```python
from build123d import *

# Parameters (mm, degrees)
ESQUISSE1_W             = 180
ESQUISSE1_H             = 70
BOSS_EXTRU_1_DEPTH      = 5
ESQUISSE3_W             = 5
ESQUISSE3_H             = 10
ESQUISSE3_W_2           = 20
ESQUISSE3_H_2           = 5
ENL_V_MAT_EXTRU_2_DEPTH = 5
ESQUISSE4_W             = 2
ESQUISSE4_H             = 30
ENL_V_MAT_EXTRU_3_DEPTH = 5


with BuildPart() as part:
    # Esquisse1 → Boss.-Extru.1 (new body)
    with BuildSketch(Plane(origin=(0, 0, 0), x_dir=(0, 0, -1), z_dir=(1, 0, 0))):
        Rectangle(ESQUISSE1_W, ESQUISSE1_H)
    extrude(amount=BOSS_EXTRU_1_DEPTH)

    # Esquisse3 → Enlèv. mat.-Extru.2 (cut)
    with BuildSketch(Plane(origin=(5, 0, 0), x_dir=(0, 0, -1), z_dir=(1, 0, 0))):
        with Locations((-87.5, 30)):
            Rectangle(ESQUISSE3_W, ESQUISSE3_H)
        with Locations((-87.5, 5)):
            Rectangle(ESQUISSE3_W, ESQUISSE3_H)
        with Locations((87.5, 30)):
            Rectangle(ESQUISSE3_W, ESQUISSE3_H)
        with Locations((87.5, 5)):
            Rectangle(ESQUISSE3_W, ESQUISSE3_H)
        with Locations((-40, 32.5)):
            Rectangle(ESQUISSE3_W_2, ESQUISSE3_H_2)
        with Locations((40, 32.5)):
            Rectangle(ESQUISSE3_W_2, ESQUISSE3_H_2)
        with Locations((0, 32.5)):
            Rectangle(ESQUISSE3_W_2, ESQUISSE3_H_2)
        with Locations((-40, -32.5)):
            Rectangle(ESQUISSE3_W_2, ESQUISSE3_H_2)
        with Locations((0, -32.5)):
            Rectangle(ESQUISSE3_W_2, ESQUISSE3_H_2)
        with Locations((40, -32.5)):
            Rectangle(ESQUISSE3_W_2, ESQUISSE3_H_2)
    extrude(amount=-ENL_V_MAT_EXTRU_2_DEPTH, mode=Mode.SUBTRACT)

    # Esquisse4 → Enlèv. mat.-Extru.3 (cut)
    with BuildSketch(Plane(origin=(5, 0, 0), x_dir=(0, 0, -1), z_dir=(1, 0, 0))):
        with Locations((32, 5)):
            Rectangle(ESQUISSE4_W, ESQUISSE4_H)
        with Locations((39, 5)):
            Rectangle(ESQUISSE4_W, ESQUISSE4_H)
        with Locations((25, 5)):
            Rectangle(ESQUISSE4_W, ESQUISSE4_H)
        with Locations((18, 5)):
            Rectangle(ESQUISSE4_W, ESQUISSE4_H)
        with Locations((11, 5)):
            Rectangle(ESQUISSE4_W, ESQUISSE4_H)
        with Locations((4, 5)):
            Rectangle(ESQUISSE4_W, ESQUISSE4_H)
        with Locations((-3, 5)):
            Rectangle(ESQUISSE4_W, ESQUISSE4_H)
        with Locations((-10, 5)):
            Rectangle(ESQUISSE4_W, ESQUISSE4_H)
        with Locations((-17, 5)):
            Rectangle(ESQUISSE4_W, ESQUISSE4_H)
        with Locations((-24, 5)):
            Rectangle(ESQUISSE4_W, ESQUISSE4_H)
    extrude(amount=-ENL_V_MAT_EXTRU_3_DEPTH, mode=Mode.SUBTRACT)


solid = part.part
```
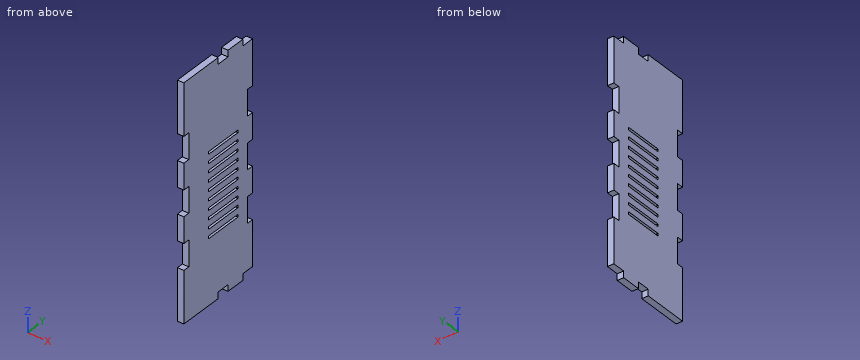
Geometry check sheet. Reference: the model listing, model coordinates, mm. Give positions to 0.01 mm unless a question says otherwise; leave off trailing zeros. Write each loop counter-clockwise with the first axis right and the second up, starting at its lowest first coordinate (ties: lowest second). Pieces come first, ordered by that corner, then holes. Notation, with made-up numbers: (-22.75, -21) -> (34.25, -21) arc R30 cw to (34.25, 3) -> close; hole circle Ø11 at (48.25, -1.75). An arc over 180 degrees is marked (long way). One line per question, with ' | ' between items.
Item 1: Depth check by flat-ended pin: pin 1 (2 mm diameter, centred on x = 2.5, z = -32, fed in from +Y); pin 2 (1.6 mm diameter, centred on x = 3.5, z = -4.5, fed in from -Y); pin 3 (2.5 mm diameter, centred on x = 3.5, y = 5.5, fed in from -Z). Enter the tip coordinate at first touch or a pass-through.
Determined:
pin 1: y = 30 | pin 2: y = -30 | pin 3: z = -85
Item 2: Scan lines: line 1 along Y through (x, z) = (1.7, -18); line 2 along Y through (x, z) = (4.4, -43); line 3 along Z through (x, y) = (0.9, 26.5). Record each from-to range of solid material in increasing order.
Determined:
line 1: -35 to -10, 20 to 35 | line 2: -30 to 30 | line 3: -85 to 85
Item 3: Sectioned sample at A-A, the plane y = 14.5. State how many separate pieces and enclosed holes the cut face has, plus the area to 3 significant figures.
Determined:
separate pieces: 11 | enclosed holes: 0 | area: 800 mm^2
Item 4: Sectioned sample at C-C, the plane z = 43.5. Record the boundary of the cut face in (x, y), plus the area to 3 significant figures.
Determined:
outline: (0, -30) -> (5, -30) -> (5, 30) -> (0, 30) -> close | area: 300 mm^2
